from build123d import *

# Parameters (mm, degrees)
SKETCH3_R          = 30
CUT_EXTRUDE1_DEPTH = 27
SKETCH4_R          = 6
CUT_EXTRUDE2_DEPTH = 112.118324226
CUT_EXTRUDE3_START = -1
SKETCH5_R          = 30
CUT_EXTRUDE3_DEPTH = 1


with BuildPart() as part:
    # Sketch2 → Revolve1 (revolve)
    with BuildSketch(Plane.XY, mode=Mode.PRIVATE) as revolve1_sk:
        Polygon((0, -14.064814815), (47, -14.064814815), (47, 11.935185185), (50, 11.935185185), (50, 14.935185185), (47, 14.935185185), (47, 17.935185185), (50, 17.935185185), (50, 20.935185185), (0, 20.935185185), align=None)
    revolve(revolve1_sk.sketch.rotate(Axis((0, 20.935185185, 0), (0, -1, 0)), 90), axis=Axis((0, 20.935185185, 0), (0, -1, 0)))

    # Sketch3 → Cut-Extrude1 (cut)
    with BuildSketch(Plane.XZ.offset(14.064814815)):
        with Locations(Location((0, 0, 0), (0, 0, 270))):
            Circle(SKETCH3_R)
    extrude(amount=-CUT_EXTRUDE1_DEPTH, mode=Mode.SUBTRACT)

    # Sketch4 → Cut-Extrude2 (cut, through all)
    with BuildSketch(Plane.XY.offset(47)):
        with Locations((0, -4.064814815)):
            Circle(SKETCH4_R)
    extrude(amount=-CUT_EXTRUDE2_DEPTH, mode=Mode.SUBTRACT)

    # Sketch5 → Cut-Extrude3 (cut)
    with BuildSketch(Plane(origin=(0, 20.935185185, 0), x_dir=(1, 0, 0), z_dir=(0, 1, 0)).offset(CUT_EXTRUDE3_START)):
        with Locations(Location((0, 0, 0), (0, 0, 90))):
            Circle(SKETCH5_R)
    extrude(amount=CUT_EXTRUDE3_DEPTH, mode=Mode.SUBTRACT)


solid = part.part
Can you work these out from the model? Positions are in its coordinate system, mm. A direction names the side the tool comes from. Coordinates: 2 decimals unless noted, no trailing zeros. Write each loop counter-clockwise with the first axis right and the second up, starting at its lowest first coordinate (ties: lowest second). Pieces come first, ordered by that corner, then holes. Notation, with made-up numbers: (33.25, 75.25) -> (56.25, 75.25) arc R9 cw to (56.25, 85.25) -> close; hole circle Ø1 at (8.5, -25.5). An arc over 180 degrees is marked (long way). Write each question's results on one line, items separated by ' | '. Start each with the question number.
Item 1: If we section it at A-A, the plane x = 0: Count the separate pieces of the cut face and the enclosed holes in it, and give its area (3 significant figures).
Item 2: If we section it at C-C, the plane z = -34.5: Write out the boundary of the cut face in (x, y).
Item 3: Thinking about a two-plate mould opening in Y: for faces 6 (the cylindrical face through (-15.02, 13.46, 47.69)), 7 (the cylindrical face through (-4.42, -0.01, 38.32)), 8 (the flat face through (33, 17.935, 34)), 9 (the flat face through (33, 11.935, 34)), which applies, released by +Y, released by -Y, zero draft, split by the parting line, or undercut?
Item 4: Please list where these lines run through material, in increasing order: probe 1 along Y at (x, z) = (0, -41.25); probe 2 along X at (y, z) = (20, 0); probe 3 along X at (y, z) = (-7.5, -27).
Item 5: I'm going to push flat-ended pins straight in: P1, Ø4, axis at x = -6, y = 15, coming from the +Z side; P2, Ø2, axis at x = -10, z = -22.5, coming from the +Y side; P3, Ø6, axis at y = 9.5, z = -33, coming from the +X side. Where does each tip first touch, or does it pass through?
Item 6: If we section it at B-B, the plane y = -5.5: Write out the boundary of the cut face in (x, z).
Item 7: On a 3-axis mill with a long thin cutter (end or side, diameter ignored), from which of +Z, -Z, +X, -X, +Y, -Y can I reach the whole of each face in a straight line? I mean faces 1 (the cylindrical face through (-14.12, -0.88, 44.83)), 2 (the cylindrical face through (-15.02, 19.46, 47.69)), 3 (the cylindrical face through (-4.42, -0.01, -38.07)), 4 (the cylindrical face through (-46.6, 16.46, -6.12)), 5 (the flat face through (0, 19.935, 0)). Say none if no direction works.
Item 8: If we section it at D-D, the plane z = 0: Write out the boundary of the cut face in (x, y).
Answer block:
1) separate pieces: 3 | enclosed holes: 0 | area: 1,240 mm²
2) outline: (-36.19, 11.94) -> (-31.92, 11.94) -> (-31.92, -14.06) -> (31.92, -14.06) -> (31.92, 11.94) -> (36.19, 11.94) -> (36.19, 14.94) -> (31.92, 14.94) -> (31.92, 17.94) -> (36.19, 17.94) -> (36.19, 20.94) -> (-36.19, 20.94) -> (-36.19, 17.94) -> (-31.92, 17.94) -> (-31.92, 14.94) -> (-36.19, 14.94) -> close; hole circle Ø12 at (0, -4.06)
3) face 6: zero draft | face 7: undercut | face 8: undercut | face 9: released by -Y
4) probe 1: -14.06 to -10.06, 1.94 to 20.94 | probe 2: -50 to -30, 30 to 50 | probe 3: -38.47 to -13.08, 13.08 to 38.47
5) P1: z = 49.84 | P2: y = 19.94 | P3: x = 39.03
6) outline: (-5.83, -46.64) -> (-5.83, -29.43) arc R30 cw to (-5.83, 29.43) -> (-5.83, 46.64) arc R47 ccw to start; (5.83, -46.64) arc R47 ccw to (5.83, 46.64) -> (5.83, 29.43) arc R30 cw to (5.83, -29.43) -> close
7) face 1: -Y | face 2: +Y, -Y | face 3: +Z, -Z | face 4: none | face 5: +Y
8) outline: (-50, 11.94) -> (-47, 11.94) -> (-47, -14.06) -> (-30, -14.06) -> (-30, 12.94) -> (30, 12.94) -> (30, -14.06) -> (47, -14.06) -> (47, 11.94) -> (50, 11.94) -> (50, 14.94) -> (47, 14.94) -> (47, 17.94) -> (50, 17.94) -> (50, 20.94) -> (30, 20.94) -> (30, 19.94) -> (-30, 19.94) -> (-30, 20.94) -> (-50, 20.94) -> (-50, 17.94) -> (-47, 17.94) -> (-47, 14.94) -> (-50, 14.94) -> close
